The listing builds one solid part. Answer for the finished solid, in the listing's coordinates (mm). A direction names the side the tool comes from. Round coordinates to 2 decimals unless told otherwise and drop trailing zeros. Loops run counter-clockwise (first coordinate to the right, second up) from the corner with the lowest first, then second, coordinate; pieces in that order, holes last. Notation, with made-up numbers: (27, -38) - (41, -38) arc R22 cw to (41, -21) - close; hole circle Ø6 at (77, -37.5). An arc over 180 degrees is marked (long way). Write item = value, one per line. Start each with the question number.
1) Given pin 1 Ø11.5 at (x, y) = (0, 0) entering from -Z; pin 2 Ø6 at (y, z) = (9, 18) entering from +X; pin 3 Ø3 at (y, z) = (-3.5, 8.5) entering from -X; pin 4 Ø5 at (y, z) = (0.5, 15) entering from +X, each flat-ended and moving along its own axis, determine where each tip first touches the part or whether it passes through.
2) Section A-A, the plane x = 0 is taken. Determine the outline of the cut face in (y, z), and give its area (3 significant figures).
3) Section C-C, the plane z = 10.75 is taken. Determine the outline of the cut face in (x, y).
4) A tool of negligible diameter and unlimited length cuts with its end or side. For faces 1 (the cylindrical face through (-2.17, 9.76, 7.48)), 2 (the cylindrical face through (11.923, 3.755, 9.352)), 3 (the cylindrical face through (-2.17, -9.76, 17.81)), from which of +Z, -Z, +X, -X, +Y, -Y can it reach the whole face along a straight path? Write none if from no direction.
5) Section B-B, the plane z = 17 is taken. Determine the outline of the cut face in (x, y), and give its area (3 significant figures).
6) Straight lines are drawn through the part: line 1 along Y through (x, z) = (0, 7.05); line 2 along Y through (x, z) = (0, 10.25); line 3 along X through (y, z) = (-6.5, 18.5). For each, find the intervals that lie inside material, in ascending order.
from build123d import *

# Parameters (mm, degrees)
SKETCH004_R     = 12.5
PAD002_DEPTH    = 8
SKETCH005_R     = 10
POCKET002_DEPTH = 3
SKETCH006_R     = 10
PAD003_DEPTH    = 8
SKETCH007_R     = 4.4
POCKET003_DEPTH = 16.001
POCKET004_DEPTH = 7
FILLET002_R     = 1.5
FILLET003_R     = 1.2


with BuildPart() as part:
    # Sketch004 → Pad002 (new body)
    with BuildSketch(Plane.XY.offset(6)):
        Circle(SKETCH004_R)
    extrude(amount=PAD002_DEPTH)

    # Sketch005 → Pocket002 (cut)
    with BuildSketch(Plane(origin=(0, 0, 6), x_dir=(1, 0, 0), z_dir=(0, 0, -1))):
        Circle(SKETCH005_R)
    extrude(amount=-POCKET002_DEPTH, mode=Mode.SUBTRACT)

    # Sketch006 → Pad003 (new body)
    with BuildSketch(Plane.XY.offset(14)):
        Circle(SKETCH006_R)
    extrude(amount=PAD003_DEPTH)

    # Sketch007 → Pocket003 (cut, through all)
    with BuildSketch(Plane.XY.offset(22)):
        Circle(SKETCH007_R)
    extrude(amount=-POCKET003_DEPTH, mode=Mode.SUBTRACT)

    # Sketch008 → Pocket004 (cut)
    with BuildSketch(Plane.XY.offset(22)):
        Polygon((4.099187, -7.1), (8.198374, 0), (4.099187, 7.1), (-4.099187, 7.1), (-8.198374, 0), (-4.099187, -7.1), align=None)
    extrude(amount=-POCKET004_DEPTH, mode=Mode.SUBTRACT)

    # Fillet002
    fillet002_edges = [part.edges().sort_by_distance(p)[0] for p in [
        (-10, 0, 22),
    ]]
    fillet(fillet002_edges, radius=FILLET002_R)

    # Fillet003
    fillet003_edges = [part.edges().sort_by_distance(p)[0] for p in [
        (-12.5, 0, 14),
        (-10, 0, 14),
    ]]
    fillet(fillet003_edges, radius=FILLET003_R)


solid = part.part
Geometry check:
q1.pin_1 = 9
q1.pin_2 = 8
q1.pin_3 = -12.34
q1.pin_4 = 12.5
q2.outline = (-12.5, 6) - (-10, 6) - (-10, 9) - (-4.4, 9) - (-4.4, 15) - (-7.1, 15) - (-7.1, 22) - (-8.5, 22) arc R1.5 ccw to (-10, 20.5) - (-10, 15.2) arc R1.2 cw to (-11.2, 14) - (-11.3, 14) arc R1.2 ccw to (-12.5, 12.8) - close; (4.4, 9) - (10, 9) - (10, 6) - (12.5, 6) - (12.5, 12.8) arc R1.2 ccw to (11.3, 14) - (11.2, 14) arc R1.2 cw to (10, 15.2) - (10, 20.5) arc R1.5 ccw to (8.5, 22) - (7.1, 22) - (7.1, 15) - (4.4, 15) - close
q2.area = 147 mm2
q3.outline = circle Ø25 at (0, 0); hole circle Ø8.8 at (0, 0)
q4.face_1 = -Z
q4.face_2 = +Z, -Z
q4.face_3 = +Z
q5.outline = circle Ø20 at (0, 0); hole (-8.2, 0) - (-4.1, -7.1) - (4.1, -7.1) - (8.2, 0) - (4.1, 7.1) - (-4.1, 7.1) - close
q5.area = 140 mm2
q6.line_1 = -12.5 to -10, 10 to 12.5
q6.line_2 = -12.5 to -4.4, 4.4 to 12.5
q6.line_3 = -7.6 to -4.45, 4.45 to 7.6
